Here's how the part is built. I have some questions about the finished solid (model axes, mm). A direction names the side the tool comes from. Coordinates: 2 decimals unless noted, no trailing zeros. Write each loop counter-clockwise with the first axis right and the second up, starting at its lowest first coordinate (ties: lowest second). Pieces come first, ordered by that corner, then holes. Notation, with made-up numbers: M -10,84.5 L 11,84.5 A16 ccw 11,93.5 Z; hole C -30.75,26 d1. An arc over 180 degrees is marked long. Use a Markdown table: item, result.
Autodesk Inventor part; units mm, degrees
ref_plane "YZ Plane" through (0, 0, 0) normal (1, 0, 0) x (0, 1, 0)
ref_plane "XZ Plane" through (0, 0, 0) normal (0, 1, 0) x (-1, 0, 0)
ref_plane "XY Plane" through (0, 0, 0) normal (0, 0, 1) x (1, 0, 0)
sketch "Sketch1" plane through (0, 0, 0) normal (0, 1, 0) x (-1, 0, 0)
  circle A0 centre (0, 0) radius 13.5
  line L0 (0, -13.5) -> (30, -13.5) construction
  line L1 (0, 13.5) -> (30, 13.5) construction
  line L2 (30, 13.5) -> (30, -13.5) construction
  line L3 (0, -13.5) -> (16, -13.5) construction
  line L4 (0, 13.5) -> (16, 13.5) construction
  line L5 (16, 13.5) -> (16, -13.5) construction
  line L6 (30, 13.5) -> (30, 9.5) construction
  line L7 (30, -13.5) -> (30, -9.5) construction
  line L8 (30, 9.5) -> (16, 9.5)
  line L9 (30, -9.5) -> (16, -9.5)
  line L10 (16, -9.5) -> (16, 9.5)
  line L11 (0, -13.5) -> (0, -16.5) construction
  line L12 (0, 13.5) -> (0, 16.5) construction
  line L13 (30, -2.5) -> (33, -2.5) construction
  line L14 (-13.5, 0) -> (-16.5, 0) construction
  line L15 (33, -2.5) -> (33, -16.5)
  line L16 (33, -16.5) -> (0, -16.5)
  line L17 (33, -2.5) -> (33, 16.5)
  line L18 (33, 16.5) -> (0, 16.5)
  line L19 (0, 16.5) -> (-16.5, 16.5)
  line L20 (-16.5, 0) -> (-16.5, 16.5)
  line L21 (0, -16.5) -> (-16.5, -16.5)
  line L22 (-16.5, -16.5) -> (-16.5, 0)
  line L23 (30, 9.5) -> (33, 9.5)
  line L24 (30, -9.5) -> (33, -9.5)
  line L25 (0, 13.5) -> (15, 13.5) construction
  line L26 (0, -13.5) -> (15, -13.5) construction
  line L27 (15, 13.5) -> (15, -13.5) construction
  line L28 (33, 9.5) -> (33, 10.5) construction
  line L29 (33, 10.5) -> (15, 10.5) construction
  line L30 (33, -9.5) -> (33, -10.5) construction
  line L31 (33, -10.5) -> (15, -10.5) construction
  line L32 (15, 10.5) -> (15, -10.5)
  line L33 (15, -10.5) -> (33, -10.5)
  line L34 (15, 10.5) -> (33, 10.5)
  dimension "d0" = 27
  dimension "d1" = 30
  dimension "d2" = 30
  dimension "d3" = 16
  dimension "d4" = 16
  dimension "d5" = 4
  dimension "d6" = 4
  dimension "d7" = 3
  dimension "d8" = 3
  dimension "d9" = 3
  dimension "d10" = 3
  dimension "d15" = 19
  dimension "d16" = 15
  dimension "d17" = 15
  dimension "d18" = 1
  dimension "d19" = 1
extrude "Extrusion3" add sketch "Sketch1" against normal blind 2 contours L34 L32 L33 L15 L16 L21 L22 L20 L19 L18 L17
extrude "Extrusion4" add sketch "Sketch1" against normal blind 10 contours L8 L10 L9 L24 L15 L33 L32 L34 L17 L23
properties part number "joystick_test_v1"
1. Suppose I cut it at B-B on y = -1.25. Write out the boundary of the cut face in (x, z).
Answers follow:
| item | result |
|---|---|
| outline | M -33,-16.5 L 16.5,-16.5 L 16.5,16.5 L -33,16.5 L -33,9.5 L -16,9.5 L -16,-9.5 L -33,-9.5 Z; hole C 0,0 d27 |
2. Suppose I cut it at C-C on z = 0. Write out the boundary of the cut face in (x, y), and give its area (3 significant figures).
Answers follow:
| item | result |
|---|---|
| outline | M -16,-10 L -15,-10 L -15,-2 L -13.5,-2 L -13.5,0 L -16,0 Z; M 13.5,-2 L 16.5,-2 L 16.5,0 L 13.5,0 Z |
| area | 19.0 mm2 |
3. I need wall thicknesses on probe 1 along Z at (x, y) = (0, -0.75); probe 2 along Y at (x, z) = (-5, 13); probe 3 along Z at (x, y) = (-30, -8.5). Which ranges of each line are inside material? Lowest first, please.
Answers follow:
| item | result |
|---|---|
| probe 1 | z = -16.5 to -13.5, 13.5 to 16.5 |
| probe 2 | y = -2 to 0 |
| probe 3 | z = -10.5 to -9.5, 9.5 to 10.5 |
4. Will these pins go through, and if not, where does the flat tip stop? pin 1 Ø5 at (x, y) = (-16, -5.5) entering from -Z; pin 2 Ø8 at (x, z) = (-23, 12.5) entering from +Y; pin 3 Ø1.5 at (x, z) = (-15.5, 12) entering from -Y.
Answers follow:
| item | result |
|---|---|
| pin 1 | stops at z = -10.5 |
| pin 2 | stops at y = 0 |
| pin 3 | stops at y = -2 |
5. We'd pull the mould along Z, two halves only. Please class faces 1 (the face through (-16, -5, 0)), 2 (the face through (-24, -6, -10.5)), 3 (the face through (-33, -3, 10)), 4 (the face through (-24, -6, 10.5)): +Z half, -Z half, draft (parallel to the pull), parting line (faces both ways), or undercut.
Answers follow:
| item | result |
|---|---|
| face 1 | undercut |
| face 2 | -Z half |
| face 3 | draft |
| face 4 | +Z half |
6. Which directions (+Z, -Z, +X, -X, +Y, -Y) give clear straight access to the entire face, cutting with the end or side of a thin tool? Please do faces 5 (the face through (-15, -6, 0)), 6 (the face through (-24, -5, -9.5)), 7 (the face through (2.93, -0.99, -13.18)).
Answers follow:
| item | result |
|---|---|
| face 5 | +Z, -Z, +X, -Y |
| face 6 | -X, +Y, -Y |
| face 7 | +Y, -Y |
7. Suppose I cut it at A-A on x = 0. Write out the boundary of the cut face in (y, z), and give its area (3 significant figures).
Answers follow:
| item | result |
|---|---|
| outline | M -2,-16.5 L 0,-16.5 L 0,-13.5 L -2,-13.5 Z; M -2,13.5 L 0,13.5 L 0,16.5 L -2,16.5 Z |
| area | 12.0 mm2 |
8. Suppose I cut it at D-D on x = -26. Write out the boundary of the cut face in (y, z), and give its area (3 significant figures).
Answers follow:
| item | result |
|---|---|
| outline | M -10,-10.5 L -2,-10.5 L -2,-16.5 L 0,-16.5 L 0,-9.5 L -10,-9.5 Z; M -10,9.5 L 0,9.5 L 0,16.5 L -2,16.5 L -2,10.5 L -10,10.5 Z |
| area | 44.0 mm2 |
